Input: part model. Units: mm. Frame: model coordinates. Give positions to 0.01 mm unless a question says otherwise; leave off trailing zeros. Loops run counter-clockwise (first coordinate to the right, second up) from the corner with the lowest first, then second, coordinate; pieces in that order, holes last. Notation, with made-up numbers: (32, 5.5) - (45, 5.5) arc R16 cw to (45, 17.5) - close; hole circle Ø8 at (67, -25). An arc over 180 degrees is marked (long way). Answer as a JSON object with one key per item and string values. Group by question number.
(1) Section query B-B (x = -10). Return loops of the section in (y, z), plus the area to 3 significant figures.
(2) Material intervals for L1, parallel to Y at x = -10, z = 1.35; L2, parallel to Y at x = 8.5, z = 0.9; L3, parallel to X at y = 2, z = 1.55, sorted ascending.
(3) Section query A-A (z = 0.9). Return loops of the section in (x, y).
(4) Section query C-C (y = -20). Return loops of the section in (x, z).
(5) Pin query (flat end, axial travel): P1, Ø4.5, axis at x = 10, y = -20, coming from the -Z side. Return the tip coordinate at first contact, or that it passes through.
(6) Mould query, pull axis Y, two halves, no side actions, for faces 1 (the cylindrical face through (-12.54, -1.05, 0.99)), 2 (the flat face through (0, 30, 1)), 3 (the flat face through (20, 0, 1)). Classes: +Y half, -Y half, draft (parallel to the pull), parting line (faces both ways), or undercut.
```python
from build123d import *

# Parameters (mm, degrees)
SKETCH_1_W        = 40
SKETCH_1_H        = 60
EXTRUDE_1_DEPTH   = 2
CHAMFER_1_SIZE    = 2
HOLE_WIZARD_M51_D = 5.5


with BuildPart() as part:
    # Эскиз1 → Бобышка-Вытянуть1 (new body)
    with BuildSketch(Plane.XY):
        Rectangle(SKETCH_1_W, SKETCH_1_H)
    extrude(amount=EXTRUDE_1_DEPTH)

    # Фаска1
    chamfer_1_edges = [part.edges().sort_by_distance(p)[0] for p in [
        (20, -30, 1),
        (-20, -30, 1),
        (-20, 30, 1),
        (20, 30, 1),
    ]]
    chamfer(chamfer_1_edges, length=CHAMFER_1_SIZE)

    # Отверстие с зазором M51 (through all)
    with Locations(Plane.XY.offset(2)):
        with Locations((-10, 20), (10, 20), (10, 0), (-10, 0), (-10, -20), (10, -20)):
            Hole(HOLE_WIZARD_M51_D / 2)


solid = part.part
```
Recorded:
{
 "1": {"outline": "(-30, 0) - (-22.75, 0) - (-22.75, 2) - (-30, 2) - close; (-17.25, 0) - (-2.75, 0) - (-2.75, 2) - (-17.25, 2) - close; (2.75, 0) - (17.25, 0) - (17.25, 2) - (2.75, 2) - close; (22.75, 0) - (30, 0) - (30, 2) - (22.75, 2) - close", "area": "87.0 mm^2"},
 "2": {"L1": "y = -30 to -22.75, -17.25 to -2.75, 2.75 to 17.25, 22.75 to 30", "L2": "y = -30 to -22.3, -17.7 to -2.3, 2.3 to 17.7, 22.3 to 30", "L3": "x = -20 to -11.89, -8.11 to 8.11, 11.89 to 20"},
 "3": {"outline": "(-20, -28) - (-18, -30) - (18, -30) - (20, -28) - (20, 28) - (18, 30) - (-18, 30) - (-20, 28) - close; hole circle Ø5.5 at (-10, -20); hole circle Ø5.5 at (-10, 0); hole circle Ø5.5 at (-10, 20); hole circle Ø5.5 at (10, -20); hole circle Ø5.5 at (10, 0); hole circle Ø5.5 at (10, 20)"},
 "4": {"outline": "(-20, 0) - (-12.75, 0) - (-12.75, 2) - (-20, 2) - close; (-7.25, 0) - (7.25, 0) - (7.25, 2) - (-7.25, 2) - close; (12.75, 0) - (20, 0) - (20, 2) - (12.75, 2) - close"},
 "5": {"P1": "passes through"},
 "6": {"face 1": "undercut", "face 2": "+Y half", "face 3": "draft"}
}
